Part model, mm, in its own coordinate system. Round coordinates to 2 decimals unless told otherwise and drop trailing zeros. Write each loop counter-clockwise with the first axis right and the second up, starting at its lowest first coordinate (ties: lowest second). Pieces come first, ordered by that corner, then holes.
1) Flat gauge pins, fed straight in: pin 1 (1 mm diameter, centred on x = 8.41, z = -6.91, fed in from -Y); pin 2 (3 mm diameter, centred on x = -5, z = 0, fed in from +Y). Where does each tip first touch, or does it go through?
2) Pull direction X, two halves, no side cores. Call faces 1 (the cylindrical face through (-6.01, 0.4, 0.65)), 2 (the flat face through (-10, 1, 0)), 3 (the flat face through (10, 1, 0)), 4 (the flat face through (0, 1, -8.5)): +X half, -X half, draft (parallel to the pull), parting line (faces both ways), or undercut.
3) Saw through at A-A on x = -5. Write the cut outline in (y, z), and give its area (3 significant figures).
4) Saw through at C-C on y = 1.35. Write the cut outline in (x, z), and give its area (3 significant figures).
5) Drill centre lines: L1, parallel to X at y = 0.4, z = 0; L2, parallel to X at y = 1.75, z = -1; L3, parallel to Z at x = -4.5, y = 1.4. Where is each one in solid material? Low to high.
6) Saw through at B-B on z = 0. Write the cut outline in (x, y), and give its area (3 significant figures).
```python
from build123d import *

# Parameters (mm, degrees)
SKETCH1_W                                      = 20
SKETCH1_H                                      = 17
BOSS_EXTRUDE1_DEPTH                            = 1.7907
F_0_80_TAPPED_HOLE1_D                          = 1.19126
CSK_FOR_M2_FLAT_HEAD_MACHINE_SCREW1_AT_2_COUNT = 2
CSK_FOR_M2_FLAT_HEAD_MACHINE_SCREW1_AT_2_PITCH = 10


with BuildPart() as part:
    # Sketch1 → Boss-Extrude1 (new body)
    with BuildSketch(Plane(origin=(0, 0, 0), x_dir=(1, 0, 0), z_dir=(0, 1, 0))):
        Rectangle(SKETCH1_W, SKETCH1_H)
    extrude(amount=BOSS_EXTRUDE1_DEPTH)

    # #0-80 Tapped Hole1 (through all)
    with Locations(Plane(origin=(0, 1.7907, 0), x_dir=(-1, 0, 0), z_dir=(0, 1, 0))):
        with Locations((-8.4125, -6.9125), (-8.4125, 6.9125), (8.4125, -6.9125), (8.4125, 6.9125)):
            Hole(F_0_80_TAPPED_HOLE1_D / 2)

    # Sketch4 → CSK for M2 Flat Head Machine Screw1 (revolve, cut)
    with BuildSketch(Plane(origin=(-5, 1.7907, 0), x_dir=(0, 0, 1), z_dir=(1, 0, 0))):
        Polygon((0, 0), (0, 1.7907), (1.2, 1.7907), (1.2, 1), (2.2, 0), align=None)
    csk_for_m2_flat_head_machine_screw1 = revolve(axis=Axis((-5, 8.1407, 0), (0, -1, 0)), mode=Mode.SUBTRACT)

    # CSK for M2 Flat Head Machine Screw1 at 2: CSK for M2 Flat Head Machine Screw1 ×2
    with Locations(*[(i * CSK_FOR_M2_FLAT_HEAD_MACHINE_SCREW1_AT_2_PITCH, 0, 0) for i in range(1, CSK_FOR_M2_FLAT_HEAD_MACHINE_SCREW1_AT_2_COUNT)]):
        add(csk_for_m2_flat_head_machine_screw1, mode=Mode.SUBTRACT)


solid = part.part
```
Completed:
1. pin 1: passes through
1. pin 2: stops at y = 1.09
2. face 1: undercut
2. face 2: -X half
2. face 3: +X half
2. face 4: draft
3. outline: (0, -8.5) - (1.79, -8.5) - (1.79, -2.2) - (0.79, -1.2) - (0, -1.2) - close; (0, 1.2) - (0.79, 1.2) - (1.79, 2.2) - (1.79, 8.5) - (0, 8.5) - close
3. area: 25.1 mm2
4. outline: (-10, -8.5) - (10, -8.5) - (10, 8.5) - (-10, 8.5) - close; hole circle Ø1.19 at (-8.41, -6.91); hole circle Ø1.19 at (-8.41, 6.91); hole circle Ø3.52 at (-5, 0); hole circle Ø3.52 at (5, 0); hole circle Ø1.19 at (8.41, -6.91); hole circle Ø1.19 at (8.41, 6.91)
4. area: 316 mm2
5. L1: x = -10 to -6.2, -3.8 to 3.8, 6.2 to 10
5. L2: x = -10 to -6.91, -3.09 to 3.09, 6.91 to 10
5. L3: z = -8.5 to -1.74, 1.74 to 8.5
6. outline: (-10, 0) - (-6.2, 0) - (-6.2, 0.79) - (-7.2, 1.79) - (-10, 1.79) - close; (-3.8, 0) - (3.8, 0) - (3.8, 0.79) - (2.8, 1.79) - (-2.8, 1.79) - (-3.8, 0.79) - close; (6.2, 0) - (10, 0) - (10, 1.79) - (7.2, 1.79) - (6.2, 0.79) - close
6. area: 25.2 mm2
